from build123d import *

# Parameters (mm, degrees)
SKETCH1_R               = 95.25
BOSS_EXTRUDE1_DEPTH     = 457.2
CUT_EXTRUDE1_DEPTH      = 457.2
CUT_EXTRUDE2_DEPTH      = 457.2
SKETCH9_W               = 179.447222202
SKETCH9_H               = 129.77242504
CUT_EXTRUDE4_DEPTH      = 11
CUT_EXTRUDE4_DEPTH_BACK = 11


with BuildPart() as part:
    # Sketch1 → Boss-Extrude1 (new body)
    with BuildSketch(Plane(origin=(0, 0, 0), x_dir=(1, 0, 0), z_dir=(0, 1, 0))):
        Circle(SKETCH1_R)
    extrude(amount=BOSS_EXTRUDE1_DEPTH)

    # Sketch2 → Cut-Extrude1 (cut)
    with BuildSketch(Plane(origin=(0, 457.2, 0), x_dir=(1, 0, 0), z_dir=(0, 1, 0))):
        with BuildLine():
            Line((89.723611101, 10), (89.723611101, 5))
            Line((89.723611101, 5), (-89.723611101, 5))
            Line((-89.723611101, 5), (-89.723611101, 10))
            Line((-89.723611101, 10), (-94.723611101, 10))
            ThreePointArc((-94.723611101, 10), (0, 95.25), (94.723611101, 10))
            Line((94.723611101, 10), (89.723611101, 10))
        make_face()
    extrude(amount=-CUT_EXTRUDE1_DEPTH, mode=Mode.SUBTRACT)

    # Sketch5 → Cut-Extrude2 (cut)
    with BuildSketch(Plane(origin=(0, 457.2, 0), x_dir=(1, 0, 0), z_dir=(0, 1, 0))):
        with BuildLine():
            Line((0, -5), (-89.723611101, -5))
            Line((-89.723611101, -5), (-89.723611101, -10))
            Line((-89.723611101, -10), (-94.723611101, -10))
            ThreePointArc((-94.723611101, -10), (0, -95.25), (94.723611101, -10))
            Line((94.723611101, -10), (89.723611101, -10))
            Line((89.723611101, -10), (89.723611101, -5))
            Line((89.723611101, -5), (0, -5))
        make_face()
    extrude(amount=-CUT_EXTRUDE2_DEPTH, mode=Mode.SUBTRACT)

    # Sketch9 → Cut-Extrude4 (cut, two sides)
    with BuildSketch(Plane.XY) as cut_extrude4_sk:
        with Locations((0, 228.6)):
            Rectangle(SKETCH9_W, SKETCH9_H)
    extrude(amount=CUT_EXTRUDE4_DEPTH, mode=Mode.SUBTRACT)
    extrude(cut_extrude4_sk.sketch, amount=-CUT_EXTRUDE4_DEPTH_BACK, mode=Mode.SUBTRACT)


solid = part.part
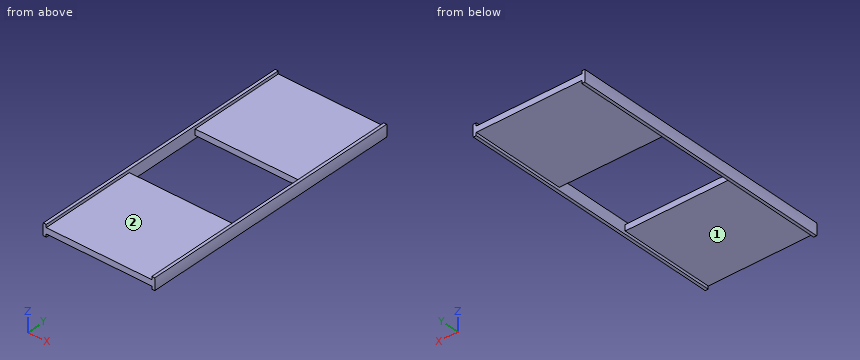
Work out the finished part from the listing and answer in its coordinate system (mm). Face numbers are marked on the shaded views. A direction names the side the tool comes from. Coordinates: 2 decimals unless noted, no trailing zeros. Order: outer loops, then holes, each group sorted by start corner. A loop starts at its lowest first (then second) coordinate and runs counter-clockwise, first axis right, second up. Notation, with made-up numbers: (46, 67.5) - (59, 67.5) arc R29 cw to (59, 105.5) - close; hole circle Ø3 at (-38.5, 21). An arc over 180 degrees is marked (long way). Put each result on its own line as item: value. Start each with the question number.
1) Find section B-B (y = 181.5). Give the vertices of the cut face in (x, z), plus the area to 3 significant figures.
2) Find section C-C (z = 1). Give the vertices of the cut face in (x, y).
3) Find the intervals of material crossed by line 1 (Y direction, x = 24, z = 0.5); line 2 (X direction, y = 376, z = 9); line 3 (X direction, y = 233.5, z = 3.75), in increasing order. Write a range as from..to.
4) Flat-ended cylindrical pins translate along their axes: pin 1 (2 mm diameter, centred on y = 174.5, z = -2, fed in from +X); pin 2 (4 mm diameter, centred on x = 55, y = 163.5, fed in from +Z); pin 3 (4 mm diameter, centred on y = 78.5, z = -3, fed in from -X). Find the tip coordinate at first contact, or state that the pin passes through.
5) Find section A-A (x = 12). Give the vertices of the cut face in (y, z).
6) Find section D-D (y = 330). Give the vertices of the cut face in (x, z).
7) For the marked faces 1 and 2, determine the directions among +Z, -Z, +X, -X, +Y, -Y from which every point of the face is accessible in a straight line to the end or side of a thin tool.
Results list:
1. outline: (-94.72, -10) - (-89.72, -10) - (-89.72, 10) - (-94.72, 10) arc R95.25 ccw to start; (89.72, -10) - (94.72, -10) arc R95.25 ccw to (94.72, 10) - (89.72, 10) - close
1. area: 214 mm^2
2. outline: (-95.24, 0) - (95.24, 0) - (95.24, 457.2) - (-95.24, 457.2) - close; hole (-89.72, 163.71) - (89.72, 163.71) - (89.72, 293.49) - (-89.72, 293.49) - close
3. line 1: y = 0..163.71, 293.49..457.2
3. line 2: x = -94.82..-89.72, 89.72..94.82
3. line 3: x = -95.18..-89.72, 89.72..95.18
4. pin 1: stops at x = 95.24
4. pin 2: stops at z = 5
4. pin 3: stops at x = -95.24
5. outline: (0, -5) - (163.71, -5) - (163.71, 5) - (0, 5) - close; (293.49, -5) - (457.2, -5) - (457.2, 5) - (293.49, 5) - close
6. outline: (-94.72, -10) - (-89.72, -10) - (-89.72, -5) - (89.72, -5) - (89.72, -10) - (94.72, -10) arc R95.25 ccw to (94.72, 10) - (89.72, 10) - (89.72, 5) - (-89.72, 5) - (-89.72, 10) - (-94.72, 10) arc R95.25 ccw to start
7. face 1: -Z, +Y, -Y
7. face 2: +Z, +Y, -Y
